Autodesk Inventor part; units mm, degrees
ref_plane "YZ Plane" through (0, 0, 0) normal (1, 0, 0) x (0, 1, 0)
ref_plane "XZ Plane" through (0, 0, 0) normal (0, 1, 0) x (-1, 0, 0)
ref_plane "XY Plane" through (0, 0, 0) normal (0, 0, 1) x (1, 0, 0)
sketch "Sketch1" plane through (0, 0, 0) normal (0, 0, 1) x (1, 0, 0)
  line L0 (176.5882, -640.9214) -> (176.5882, 349.6786)
  line L1 (176.5882, 349.6786) -> (-77.4118, 349.6786)
  line L2 (-77.4118, 349.6786) -> (-77.4118, -640.9214)
  line L3 (100.3882, -640.9214) -> (100.3882, -564.7214)
  line L4 (100.3882, -564.7214) -> (176.5882, -564.7214)
  line L5 (176.5882, -475.8214) -> (100.3882, -475.8214)
  line L6 (100.3882, -475.8214) -> (100.3882, -399.6214)
  line L7 (100.3882, -399.6214) -> (176.5882, -399.6214)
  line L8 (176.5882, -399.6214) -> (176.5882, -475.8214)
  line L9 (176.5882, -94.8214) -> (100.3882, -94.8214)
  line L10 (100.3882, -94.8214) -> (100.3882, 70.2786)
  line L11 (100.3882, 70.2786) -> (176.5882, 70.2786)
  line L12 (176.5882, 70.2786) -> (176.5882, -94.8214)
  line L13 (176.5882, 349.6786) -> (100.3882, 349.6786)
  line L14 (100.3882, 349.6786) -> (100.3882, 273.4786)
  line L15 (100.3882, 273.4786) -> (176.5882, 273.4786)
  line L16 (176.5882, 273.4786) -> (176.5882, 349.6786)
  line L17 (-77.4118, 275.381) -> (-77.4118, 369.0362)
  line L18 (-77.4118, -16.7496) -> (-77.4118, 88.2844)
  line L19 (-77.4118, -379.8866) -> (-77.4118, -294.668)
  line L20 (-77.4118, -640.9214) -> (-1.2118, -640.9214)
  line L21 (-1.2118, -640.9214) -> (-1.2118, -564.7214)
  line L22 (-1.2118, -564.7214) -> (-77.4118, -564.7214)
  line L23 (-77.4118, -564.7214) -> (-77.4118, -640.9214)
  line L24 (-77.4118, -259.9214) -> (-1.2118, -259.9214)
  line L25 (-1.2118, -259.9214) -> (-1.2118, -336.1214)
  line L26 (-1.2118, -336.1214) -> (-77.4118, -336.1214)
  line L27 (-77.4118, -336.1214) -> (-77.4118, -259.9214)
  line L28 (-77.4118, -5.9214) -> (-1.2118, -5.9214)
  line L29 (-1.2118, -5.9214) -> (-1.2118, 70.2786)
  line L30 (-1.2118, 70.2786) -> (-77.4118, 70.2786)
  line L31 (-77.4118, 70.2786) -> (-77.4118, -5.9214)
  line L32 (-77.4118, 349.6786) -> (-1.2118, 349.6786)
  line L33 (-1.2118, 349.6786) -> (-1.2118, 273.4786)
  line L34 (-1.2118, 273.4786) -> (-77.4118, 273.4786)
  line L35 (-77.4118, 273.4786) -> (-77.4118, 349.6786)
  line L36 (100.3882, -640.9214) -> (100.3882, -666.3214)
  line L37 (100.3882, -666.3214) -> (-1.2118, -666.3214)
  line L38 (-1.2118, -666.3214) -> (-1.2118, -640.9214)
  point P0 (0, 0)
  point P1 (49.5882, -323.4214)
  point P2 (-64.7118, -437.7214)
  point P3 (-64.7118, -132.9214)
  point P4 (163.8882, 171.8786)
  point P5 (-64.7118, 171.8786)
  point P6 (163.8882, -196.4214)
  point P7 (163.8882, -513.9214)
  point P8 (49.5882, -653.6214)
  point P9 (49.5882, 6.7786)
  dimension "d0" = 254
  dimension "d1" = 990.6
  dimension "d2" = 76.2
  dimension "d3" = 76.2
  dimension "d4" = 76.2
  dimension "d5" = 76.2
  dimension "d6" = 88.9
  dimension "d7" = 304.8
  dimension "d8" = 203.2
  dimension "d9" = 76.2
  dimension "d10" = 76.2
  dimension "d11" = 76.2
  dimension "d14" = 76.2
  dimension "d15" = 76.2
  dimension "d16" = 76.2
  dimension "d17" = 76.2
  dimension "d18" = 63.5
  dimension "d19" = 76.2
  dimension "d20" = 76.2
  dimension "d21" = 203.2
  dimension "d22" = 76.2
  dimension "d23" = 76.2
  dimension "d24" = 12.7
  dimension "d25" = 12.7
  dimension "d26" = 101.6
  dimension "d27" = 101.6
  dimension "d28" = 127
  dimension "d29" = 12.7
  dimension "d30" = 12.7
  dimension "d31" = 127
  dimension "d32" = 101.6
  dimension "d33" = 12.7
  dimension "d34" = 12.7
  dimension "d35" = 101.6
  dimension "d36" = 38.1
  dimension "d37" = 25.4
  dimension "d38" = 101.6
  dimension "d46" = 12.7
extrude "Extrusion1" add sketch "Sketch1" against normal blind 3.175 contours L4 L3 L36 L37 L38 L21 L22 L2 L26 L25 L24 L28 L29 L30 L34 L33 L1 L14 L15 L0 L11 L10 L9 L7 L6 L5
hole "Hole1" at (49.5882, -323.4214, 0) at (-64.7118, -437.7214, 0) at (-64.7118, -132.9214, 0) at (163.8882, 171.8786, 0) at (-64.7118, 171.8786, 0) at (163.8882, -196.4214, 0) at (163.8882, -513.9214, 0) at (49.5882, -653.6214, 0) at (49.5882, 6.7786, 0) direction (0, 0, -1) diameter 6.35 depth 25.4 tip angle 118
properties part number "tower walls"
Geometry check sheet. Reference: the model listing, model coordinates, mm. Round coordinates to 2 decimals unless told otherwise and drop trailing zeros. Loops run counter-clockwise (first coordinate to the right, second up) from the corner with the lowest first, then second, coordinate; pieces in that order, holes last.
Item 1: Cross-section at A-A on x = 111.5. Record the boundary of the cut face in (y, z) (3 decimals).
Item 2: Cross-section at B-B on y = -286.5. Record the boundary of the cut face in (x, z) (3 decimals).
Item 3: Gauge pin test, flat ends, axial feed: pin 1 (1 mm diameter, centred on x = 129, z = -2.5, fed in from +Y); pin 2 (1.6 mm diameter, centred on y = 33.5, z = -2, fed in from -X); pin 3 (1 mm diameter, centred on y = 35, z = -1.5, fed in from +X). Record the tip position at first contact, or that the pin passes through.
Item 4: Thickness scan on line 1 (Y direction, x = 160, z = -0.55); line 2 (Y direction, x = -64, z = -0.2); line 3 (Y direction, x = -60, z = -2). Record the ranges inside material, lowest first.
Item 5: Cross-section at C-C on z = -1.5. Count the separate pieces of the cut face and the enclosed holes in it, then the cut area to 3 significant figures.
Answer sheet:
1. outline: (-564.721, -3.175) - (-475.821, -3.175) - (-475.821, 0) - (-564.721, 0) - close; (-399.621, -3.175) - (-94.821, -3.175) - (-94.821, 0) - (-399.621, 0) - close; (70.279, -3.175) - (273.479, -3.175) - (273.479, 0) - (70.279, 0) - close
2. outline: (-1.212, -3.175) - (176.588, -3.175) - (176.588, 0) - (-1.212, 0) - close
3. pin 1: stops at y = 273.48
3. pin 2: stops at x = -1.21
3. pin 3: stops at x = 100.39
4. line 1: y = -564.72 to -475.82, -399.62 to -94.82, 70.28 to 273.48
4. line 2: y = -564.72 to -440.82, -434.63 to -336.12, -259.92 to -136.02, -129.83 to -5.92, 70.28 to 168.78, 174.97 to 273.48
4. line 3: y = -564.72 to -336.12, -259.92 to -5.92, 70.28 to 273.48
5. separate pieces: 1
5. enclosed holes: 9
5. area: 201,000 mm2
